Verification items for this drawing (mm, ordinates from the low corner). Coordinates: 2 decimals unless noted, no trailing zeros. Order: outer loops, then holes, each group sorted by start corner. A loop starts at its lowest first (then second) coordinate and runs counter-clockwise, first axis right, second up. Notation, with made-up numbers: M 28.25,-16 L 47.25,-16 A19 cw 47.25,19 Z; hole C -27.5,88.25 d4. An arc over 180 degrees is marked long. Write item = value, one per line.
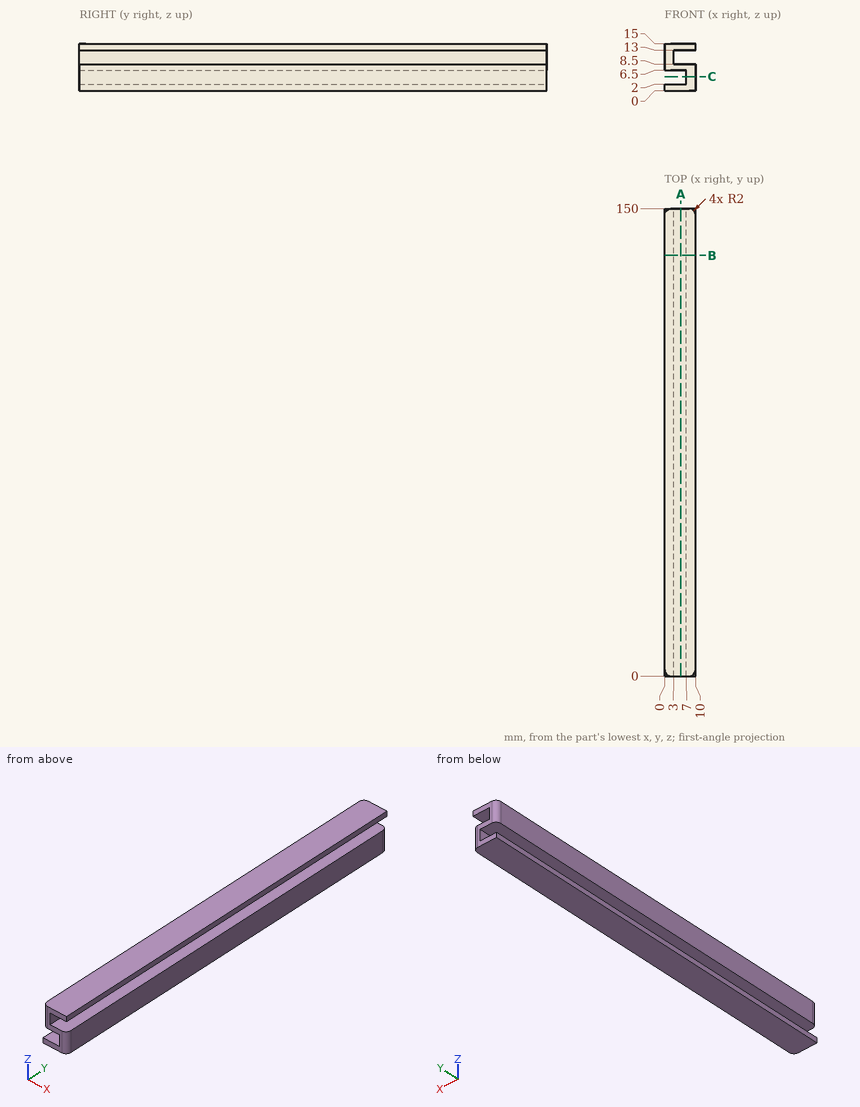
Item 1: Scan lines: L1, parallel to Z at x = 4.5, y = 15; L2, parallel to Z at x = 8.75, y = 118; L3, parallel to Z at x = 2.75, y = 74. Record each from-to range of solid material in increasing order. Write a range as from..to.
Report:
L1 = 0..2, 6.5..8.5, 13..15
L2 = 0..8.5, 13..15
L3 = 0..2, 6.5..15
Item 2: Sectioned sample at B-B, the plane y = 135. Enter the section's corners in (x, z).
Report:
outline = M 0,0 L 10,0 L 10,8.5 L 3,8.5 L 3,13 L 10,13 L 10,15 L 0,15 L 0,6.5 L 7,6.5 L 7,2 L 0,2 Z
Item 3: Sectioned sample at C-C, the plane z = 4.5. Enter the section's corners in (x, y).
Report:
outline = M 7,0 L 8,0 A2 ccw 10,2 L 10,148 A2 ccw 8,150 L 7,150 Z
Item 4: Sectioned sample at A-A, the plane x = 5.25. Enter the section's corners in (y, z), then the cut area to 3 significant figures.
Report:
outline = M 0,0 L 150,0 L 150,2 L 0,2 Z; M 0,6.5 L 150,6.5 L 150,8.5 L 0,8.5 Z; M 0,13 L 150,13 L 150,15 L 0,15 Z
area = 900 mm^2
